```python
from build123d import *

# Parameters (mm, degrees)
BOSS_EXTRUDE1_DEPTH      = 36.650000106
BOSS_EXTRUDE3_DEPTH      = 6.35
S_0_348_DIAMETER_HOLE1_D = 8.8392


with BuildPart() as part:
    # Sketch1 → Boss-Extrude1 (new body)
    with BuildSketch(Plane(origin=(0, 0, 0), x_dir=(1, 0, 0), z_dir=(0, 1, 0))):
        Polygon((12.954, 19.05), (31.75, 19.05), (31.75, 12.954), (19.05, 12.954), (19.05, 6.35), (31.75, 6.35), (31.75, 0), (3.574718809, -10.254963696), (-12.592782584, 1.065642654), (0, 19.05), (6.35, 19.05), (6.35, 6.35), (12.954, 6.35), align=None)
    extrude(amount=BOSS_EXTRUDE1_DEPTH)

    # Sketch8 → Boss-Extrude3 (add)
    with BuildSketch(Plane.XZ):
        Polygon((6.35, -19.05), (12.954, -19.05), (31.75, -19.05), (31.75, -12.954), (31.75, -6.35), (31.75, 0), (3.574718809, 10.254963696), (-12.592782584, -1.065642654), (0, -19.05), align=None)
    extrude(amount=BOSS_EXTRUDE3_DEPTH)

    # S (0.348) Diameter Hole1 (through all)
    with Locations(Plane(origin=(0, 36.650000106, 0), x_dir=(1, 0, 0), z_dir=(0, 1, 0))):
        with Locations((-0.939868465, 2.208486712)):
            Hole(S_0_348_DIAMETER_HOLE1_D / 2)


solid = part.part
```
CAD build for the part. Positions are in the model's coordinates, mm. A direction names the side the tool comes from. Round coordinates to 2 decimals unless told otherwise and drop trailing zeros. Order: outer loops, then holes, each group sorted by start corner. A loop starts at its lowest first (then second) coordinate and runs counter-clockwise, first axis right, second up. Notation, with made-up numbers: (35, 28.25) - (65, 28.25) arc R28 cw to (65, 61.25) - close; hole circle Ø8 at (-31, -31). An arc over 180 degrees is marked (long way). Answer in a Markdown table with one row per item. Add a question column.
(1) Band-saw the part on D-D on x = 20.5. List the corners of the cut face in (y, z).
(2) Band-saw the part on A-A on x = -1.5. List the corners of the cut face in (y, z).
(3) 3-axis set-ups, long thin cutter, end or side, ignore diameter. For faces 1 (the face through (-6.385, 15.451, -9.932)), 2 (the face through (6.35, 18, -13)), 3 (the face through (25, 18, -12.954)): which of +Z, -Z, +X, -X, +Y, -Y reach the whole face in a straight line?
(4) Drop flat-ended pins along their axis: pin 1 Ø4 at (y, z) = (24, -11) entering from -X; pin 2 Ø5 at (y, z) = (14, -7.5) entering from +X; pin 3 Ø2 at (x, z) = (11, -13.5) entering from +Y; pin 4 Ø14 at (x, y) = (25.5, 12) entering from +Z. Give the stop position or say it passes through.
(5) Band-saw the part on C-C on z = -9.75. List the corners of the cut face in (x, y), and give its area (3 significant figures).
(6) Band-saw the part on B-B on y = 33. List the corners of the cut face in (x, z), and give its area (3 significant figures).
(7) Probe L1, parallel to Y at x = 10, z = -10.5; L2, parallel to X at y = 19, z = -15.75; L3, parallel to X at y = 19, z = -16.5. List the from-to ranges inside material, lowest first. Write a range as [from, to].
(8) Mould opens along Z. For faces 4 (the face through (-0.36, 14.85, -6.59)), 5 (the face through (-4.4, 15.45, 4.67)), 6 (the face through (31.75, 15, -14)) say: +Z half, -Z half, draft (parallel to the pull), parting line (faces both ways), or undercut.
Data:
| question | item | result |
|---|---|---|
| 1 | outline | (-6.35, -19.05) - (36.65, -19.05) - (36.65, -12.95) - (0, -12.95) - (0, -6.35) - (36.65, -6.35) - (36.65, 4.09) - (-6.35, 4.09) - close |
| 2 | outline | (-6.35, -16.91) - (36.65, -16.91) - (36.65, -6.59) - (-6.35, -6.59) - close; (-6.35, 2.18) - (36.65, 2.18) - (36.65, 6.7) - (-6.35, 6.7) - close |
| 3 | face 1 | -Z, -X, +Y, -Y |
| 3 | face 2 | -Z, +Y |
| 3 | face 3 | +X, +Y |
| 4 | pin 1 | stops at x = -7.04 |
| 4 | pin 2 | stops at x = 31.75 |
| 4 | pin 3 | stops at y = 0 |
| 4 | pin 4 | stops at z = 4.82 |
| 5 | outline | (-6.51, -6.35) - (31.75, -6.35) - (31.75, 0) - (19.05, 0) - (19.05, 36.65) - (12.95, 36.65) - (12.95, 0) - (6.35, 0) - (6.35, 36.65) - (-6.51, 36.65) - close |
| 5 | area | 938 mm^2 |
| 6 | outline | (-12.59, -1.07) - (0, -19.05) - (6.35, -19.05) - (6.35, -6.35) - (12.95, -6.35) - (12.95, -19.05) - (31.75, -19.05) - (31.75, -12.95) - (19.05, -12.95) - (19.05, -6.35) - (31.75, -6.35) - (31.75, 0) - (3.57, 10.25) - close; hole circle Ø8.84 at (-0.94, -2.21) |
| 6 | area | 721 mm^2 |
| 7 | L1 | y = [-6.35, 0] |
| 7 | L2 | x = [-2.31, 6.35], [12.95, 31.75] |
| 7 | L3 | x = [-1.79, 6.35], [12.95, 31.75] |
| 8 | face 4 | undercut |
| 8 | face 5 | +Z half |
| 8 | face 6 | draft |
